Verification items for the finished model (mm, model axes). Face numbers are marked on the shaded views. A direction names the side the tool comes from. Coordinates: 2 decimals unless noted, no trailing zeros. Write each loop counter-clockwise with the first axis right and the second up, starting at its lowest first coordinate (ties: lowest second). Pieces come first, ordered by that corner, then holes. Notation, with made-up numbers: (18.5, -34) -> (41.5, -34) arc R38 cw to (41.5, 5) -> close; hole circle Ø2 at (19, 59.5). An arc over 180 degrees is marked (long way). Use CSV: the item, a comma, the result in double quotes.
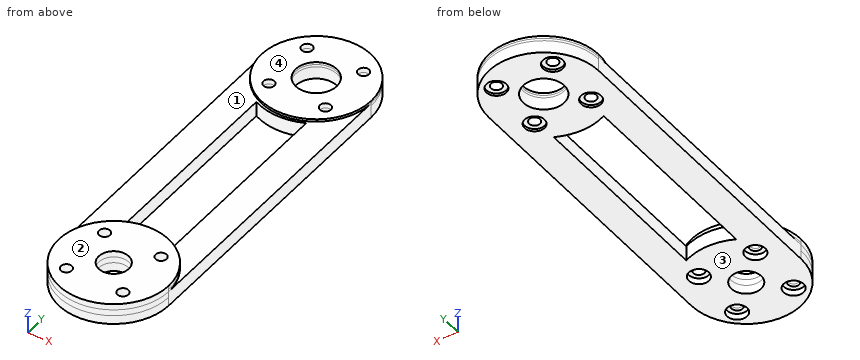
```python
from build123d import *

# Parameters (mm, degrees)
BOSS_EXTRUDE1_DEPTH           = 3
BOSS_EXTRUDE2_START           = -0.5
SKETCH1_3_R                   = 11
BOSS_EXTRUDE2_DEPTH           = 0.5
SKETCH2_R                     = 4.1
SKETCH2_R_2                   = 1.1000000000000099
CUT_EXTRUDE1_DEPTH            = 3.5
SKETCH2_3_R                   = 2.000000000000007
CUT_EXTRUDE2_DEPTH            = 0.5
CIRPATTERN2_COUNT             = 4
BOSS_EXTRUDE3_START           = -1.225
SKETCH1_5_R                   = 11
BOSS_EXTRUDE3_DEPTH           = 1.225
SKETCH3_R                     = 3.0000000000000004
SKETCH3_R_2                   = 1.1
CUT_EXTRUDE3_DEPTH            = 4.225
SKETCH3_3_R                   = 2.0000000000000027
CUT_EXTRUDE4_DEPTH            = 1.225
CIRPATTERN3_COUNT             = 4
BODY_MOVE_COPY1_START         = -3
BODY_MOVE_COPY1_OUTLINE_R     = 2
BODY_MOVE_COPY1_OUTLINE_R_2   = 3
BODY_MOVE_COPY1_OUTLINE_R_3   = 4.1
BODY_MOVE_COPY1_DEPTH         = 3
BODY_MOVE_COPY1_START_2       = -2.5
BODY_MOVE_COPY1_2_OUTLINE_R   = 2
BODY_MOVE_COPY1_2_OUTLINE_R_2 = 1.1
BODY_MOVE_COPY1_2_DEPTH       = 2
BODY_MOVE_COPY1_START_3       = -1.775
BODY_MOVE_COPY1_3_OUTLINE_R   = 2
BODY_MOVE_COPY1_3_OUTLINE_R_2 = 1.1
BODY_MOVE_COPY1_3_DEPTH       = 0.55
BODY_MOVE_COPY1_START_4       = 0.5
BODY_MOVE_COPY1_4_OUTLINE_R   = 4.1
BODY_MOVE_COPY1_4_OUTLINE_R_2 = 1.1
BODY_MOVE_COPY1_4_DEPTH       = 2.5
BODY_MOVE_COPY1_START_5       = 1.225
BODY_MOVE_COPY1_5_OUTLINE_R   = 11
BODY_MOVE_COPY1_5_OUTLINE_R_2 = 3
BODY_MOVE_COPY1_5_OUTLINE_R_3 = 1.1
BODY_MOVE_COPY1_5_DEPTH       = 1.775
BODY_MOVE_COPY1_6_DEPTH       = 0.5


# Read off the part's stored shape, not the designer's step: Body-Move/Copy1
with BuildPart() as part:
    # Sketch1 → Boss-Extrude1 (new body)
    with BuildSketch(Plane.XY):
        with BuildLine():
            Line((-11.000000000000004, 30), (-11, -30))
            ThreePointArc((-11, -30), (-2.02e-15, -41), (11, -30.000000000000004))
            Line((11, -30), (10.999999999999996, 30))
            ThreePointArc((10.999999999999996, 30), (-5.6e-16, 41), (-11.000000000000004, 30.000000000000007))
        make_face()
        with BuildLine():
            ThreePointArc((4.999999999999998, -19.643842411396), (2.89e-15, -18.49999999999999), (-4.999999999999995, -19.643842411396))
            Line((-4.999999999999993, -19.643842411396008), (-5.0000000000000036, 19.643842411396008))
            ThreePointArc((-5.000000000000004, 19.643842411396008), (1.78e-15, 18.5), (5.000000000000006, 19.643842411396008))
            Line((5.0000000000000036, 19.643842411396008), (4.999999999999998, -19.643842411396008))
        make_face(mode=Mode.SUBTRACT)
    extrude(amount=BOSS_EXTRUDE1_DEPTH)

    # Sketch1<3> → Boss-Extrude2 (add)
    with BuildSketch(Plane.XY.offset(BOSS_EXTRUDE2_START)):
        with Locations((-3.67e-15, 30)):
            Circle(SKETCH1_3_R)
    extrude(amount=BOSS_EXTRUDE2_DEPTH)

    # Sketch2 → Cut-Extrude1 (cut)
    with BuildSketch(Plane.XY.offset(3)):
        with Locations((-3.67e-15, 30)):
            Circle(SKETCH2_R)
        with Locations((5.6568542494923415, 35.656854249492405)):
            Circle(SKETCH2_R_2)
    cut_extrude1 = extrude(amount=-CUT_EXTRUDE1_DEPTH, mode=Mode.SUBTRACT)

    # Sketch2<3> → Cut-Extrude2 (cut)
    with BuildSketch(Plane.XY.offset(3)):
        with Locations((5.6568542494923415, 35.656854249492405)):
            Circle(SKETCH2_3_R)
    cut_extrude2 = extrude(amount=-CUT_EXTRUDE2_DEPTH, mode=Mode.SUBTRACT)

    # CirPattern2: Cut-Extrude1, Cut-Extrude2 ×4 about axis
    cirpattern2_axis = Axis((-1.339e-14, 30.00000000000001, 0), (0, 0, 1))
    add([cut_extrude1.rotate(cirpattern2_axis, i * 360 / CIRPATTERN2_COUNT) for i in range(1, CIRPATTERN2_COUNT)], mode=Mode.SUBTRACT)
    add([cut_extrude2.rotate(cirpattern2_axis, i * 360 / CIRPATTERN2_COUNT) for i in range(1, CIRPATTERN2_COUNT)], mode=Mode.SUBTRACT)

    # Sketch1<5> → Boss-Extrude3 (add)
    with BuildSketch(Plane.XY.offset(BOSS_EXTRUDE3_START)):
        with Locations((0, -30)):
            Circle(SKETCH1_5_R)
    extrude(amount=BOSS_EXTRUDE3_DEPTH)

    # Sketch3 → Cut-Extrude3 (cut)
    with BuildSketch(Plane.XY.offset(3)):
        with Locations((0, -30)):
            Circle(SKETCH3_R)
        with Locations((5.656854249492389, -24.34314575050763)):
            Circle(SKETCH3_R_2)
    cut_extrude3 = extrude(amount=-CUT_EXTRUDE3_DEPTH, mode=Mode.SUBTRACT)

    # Sketch3<3> → Cut-Extrude4 (cut)
    with BuildSketch(Plane.XY.offset(3)):
        with Locations((5.656854249492389, -24.34314575050763)):
            Circle(SKETCH3_3_R)
    cut_extrude4 = extrude(amount=-CUT_EXTRUDE4_DEPTH, mode=Mode.SUBTRACT)

    # CirPattern3: Cut-Extrude3, Cut-Extrude4 ×4 about axis
    cirpattern3_axis = Axis((-9.49e-15, -29.99999999999999, 0), (0, 0, 1))
    add([cut_extrude3.rotate(cirpattern3_axis, i * 360 / CIRPATTERN3_COUNT) for i in range(1, CIRPATTERN3_COUNT)], mode=Mode.SUBTRACT)
    add([cut_extrude4.rotate(cirpattern3_axis, i * 360 / CIRPATTERN3_COUNT) for i in range(1, CIRPATTERN3_COUNT)], mode=Mode.SUBTRACT)

    # Body-Move/Copy1 outline → Body-Move/Copy1 (add)
    with BuildSketch(Plane.XY.offset(BODY_MOVE_COPY1_START)):
        with BuildLine():
            Line((-11, 30), (-11, -30))
            ThreePointArc((-11, -30), (0, -41), (11, -30))
            Line((11, -30), (11, 30))
            ThreePointArc((11, 30), (0, 41), (-11, 30))
        make_face()
        with BuildLine():
            Line((-5, -19.643842411), (-5, 19.643842411))
            ThreePointArc((-5, 19.643842411), (0, 18.5), (5, 19.643842411))
            Line((5, 19.643842411), (5, -19.643842411))
            ThreePointArc((5, -19.643842411), (0, -18.5), (-5, -19.643842411))
        make_face(mode=Mode.SUBTRACT)
        with Locations((5.656854249, -24.343145751)):
            Circle(BODY_MOVE_COPY1_OUTLINE_R, mode=Mode.SUBTRACT)
        with Locations((-5.656854249, -35.656854249)):
            Circle(BODY_MOVE_COPY1_OUTLINE_R, mode=Mode.SUBTRACT)
        with Locations((-5.656854249, -24.343145751)):
            Circle(BODY_MOVE_COPY1_OUTLINE_R, mode=Mode.SUBTRACT)
        with Locations((0, -30)):
            Circle(BODY_MOVE_COPY1_OUTLINE_R_2, mode=Mode.SUBTRACT)
        with Locations((5.656854249, -35.656854249)):
            Circle(BODY_MOVE_COPY1_OUTLINE_R, mode=Mode.SUBTRACT)
        with Locations((5.656854249, 35.656854249)):
            Circle(BODY_MOVE_COPY1_OUTLINE_R, mode=Mode.SUBTRACT)
        with Locations((-5.656854249, 24.343145751)):
            Circle(BODY_MOVE_COPY1_OUTLINE_R, mode=Mode.SUBTRACT)
        with Locations((-5.656854249, 35.656854249)):
            Circle(BODY_MOVE_COPY1_OUTLINE_R, mode=Mode.SUBTRACT)
        with Locations((0, 30)):
            Circle(BODY_MOVE_COPY1_OUTLINE_R_3, mode=Mode.SUBTRACT)
        with Locations((5.656854249, 24.343145751)):
            Circle(BODY_MOVE_COPY1_OUTLINE_R, mode=Mode.SUBTRACT)
    extrude(amount=BODY_MOVE_COPY1_DEPTH)

    # Body-Move_Copy1 2 outline → Body-Move_Copy1 2 (add)
    # profile 1 of 4: a face of its own
    with BuildSketch(Plane.XY.offset(BODY_MOVE_COPY1_START_2)):
        with Locations((5.656854249, 35.656854249)):
            Circle(BODY_MOVE_COPY1_2_OUTLINE_R)
        with Locations((5.656854249, 35.656854249)):
            Circle(BODY_MOVE_COPY1_2_OUTLINE_R_2, mode=Mode.SUBTRACT)
    # profile 2 of 4: a face of its own
    with BuildSketch(Plane.XY.offset(BODY_MOVE_COPY1_START_2)):
        with Locations((5.656854249, 24.343145751)):
            Circle(BODY_MOVE_COPY1_2_OUTLINE_R)
        with Locations((5.656854249, 24.343145751)):
            Circle(BODY_MOVE_COPY1_2_OUTLINE_R_2, mode=Mode.SUBTRACT)
    # profile 3 of 4: a face of its own
    with BuildSketch(Plane.XY.offset(BODY_MOVE_COPY1_START_2)):
        with Locations((-5.656854249, 35.656854249)):
            Circle(BODY_MOVE_COPY1_2_OUTLINE_R)
        with Locations((-5.656854249, 35.656854249)):
            Circle(BODY_MOVE_COPY1_2_OUTLINE_R_2, mode=Mode.SUBTRACT)
    # profile 4 of 4: a face of its own
    with BuildSketch(Plane.XY.offset(BODY_MOVE_COPY1_START_2)):
        with Locations((-5.656854249, 24.343145751)):
            Circle(BODY_MOVE_COPY1_2_OUTLINE_R)
        with Locations((-5.656854249, 24.343145751)):
            Circle(BODY_MOVE_COPY1_2_OUTLINE_R_2, mode=Mode.SUBTRACT)
    extrude(amount=BODY_MOVE_COPY1_2_DEPTH)

    # Body-Move_Copy1 3 outline → Body-Move_Copy1 3 (add)
    # profile 1 of 4: a face of its own
    with BuildSketch(Plane.XY.offset(BODY_MOVE_COPY1_START_3)):
        with Locations((5.656854249, -24.343145751)):
            Circle(BODY_MOVE_COPY1_3_OUTLINE_R)
        with Locations((5.656854249, -24.343145751)):
            Circle(BODY_MOVE_COPY1_3_OUTLINE_R_2, mode=Mode.SUBTRACT)
    # profile 2 of 4: a face of its own
    with BuildSketch(Plane.XY.offset(BODY_MOVE_COPY1_START_3)):
        with Locations((5.656854249, -35.656854249)):
            Circle(BODY_MOVE_COPY1_3_OUTLINE_R)
        with Locations((5.656854249, -35.656854249)):
            Circle(BODY_MOVE_COPY1_3_OUTLINE_R_2, mode=Mode.SUBTRACT)
    # profile 3 of 4: a face of its own
    with BuildSketch(Plane.XY.offset(BODY_MOVE_COPY1_START_3)):
        with Locations((-5.656854249, -24.343145751)):
            Circle(BODY_MOVE_COPY1_3_OUTLINE_R)
        with Locations((-5.656854249, -24.343145751)):
            Circle(BODY_MOVE_COPY1_3_OUTLINE_R_2, mode=Mode.SUBTRACT)
    # profile 4 of 4: a face of its own
    with BuildSketch(Plane.XY.offset(BODY_MOVE_COPY1_START_3)):
        with Locations((-5.656854249, -35.656854249)):
            Circle(BODY_MOVE_COPY1_3_OUTLINE_R)
        with Locations((-5.656854249, -35.656854249)):
            Circle(BODY_MOVE_COPY1_3_OUTLINE_R_2, mode=Mode.SUBTRACT)
    extrude(amount=BODY_MOVE_COPY1_3_DEPTH)

    # Body-Move_Copy1 4 outline → Body-Move_Copy1 4 (cut)
    with BuildSketch(Plane.XY.offset(BODY_MOVE_COPY1_START_4)):
        with BuildLine():
            ThreePointArc((-11, -30), (0, -19), (11, -30))
            Line((11, -30), (11, 30))
            ThreePointArc((11, 30), (0, 41), (-11, 30))
            Line((-11, 30), (-11, -30))
        make_face()
        with BuildLine():
            Line((-5, -19.643842411), (-5, 19.643842411))
            ThreePointArc((-5, 19.643842411), (0, 18.5), (5, 19.643842411))
            Line((5, 19.643842411), (5, -19.643842411))
            ThreePointArc((5, -19.643842411), (0, -18.5), (-5, -19.643842411))
        make_face(mode=Mode.SUBTRACT)
        with Locations((0, 30)):
            Circle(BODY_MOVE_COPY1_4_OUTLINE_R, mode=Mode.SUBTRACT)
        with Locations((5.656854249, 35.656854249)):
            Circle(BODY_MOVE_COPY1_4_OUTLINE_R_2, mode=Mode.SUBTRACT)
        with Locations((-5.656854249, 24.343145751)):
            Circle(BODY_MOVE_COPY1_4_OUTLINE_R_2, mode=Mode.SUBTRACT)
        with Locations((-5.656854249, 35.656854249)):
            Circle(BODY_MOVE_COPY1_4_OUTLINE_R_2, mode=Mode.SUBTRACT)
        with Locations((5.656854249, 24.343145751)):
            Circle(BODY_MOVE_COPY1_4_OUTLINE_R_2, mode=Mode.SUBTRACT)
    extrude(amount=BODY_MOVE_COPY1_4_DEPTH, mode=Mode.SUBTRACT)

    # Body-Move_Copy1 5 outline → Body-Move_Copy1 5 (cut)
    with BuildSketch(Plane.XY.offset(BODY_MOVE_COPY1_START_5)):
        with Locations((0, -30)):
            Circle(BODY_MOVE_COPY1_5_OUTLINE_R)
        with Locations((0, -30)):
            Circle(BODY_MOVE_COPY1_5_OUTLINE_R_2, mode=Mode.SUBTRACT)
        with Locations((-5.656854249, -35.656854249)):
            Circle(BODY_MOVE_COPY1_5_OUTLINE_R_3, mode=Mode.SUBTRACT)
        with Locations((-5.656854249, -24.343145751)):
            Circle(BODY_MOVE_COPY1_5_OUTLINE_R_3, mode=Mode.SUBTRACT)
        with Locations((5.656854249, -35.656854249)):
            Circle(BODY_MOVE_COPY1_5_OUTLINE_R_3, mode=Mode.SUBTRACT)
        with Locations((5.656854249, -24.343145751)):
            Circle(BODY_MOVE_COPY1_5_OUTLINE_R_3, mode=Mode.SUBTRACT)
    extrude(amount=BODY_MOVE_COPY1_5_DEPTH, mode=Mode.SUBTRACT)

    # Body-Move_Copy1 6 outline → Body-Move_Copy1 6 (cut)
    with BuildSketch(Plane.XY):
        with BuildLine():
            ThreePointArc((-11, -30), (0, -19), (11, -30))
            Line((11, -30), (11, 30))
            ThreePointArc((11, 30), (0, 19), (-11, 30))
            Line((-11, 30), (-11, -30))
        make_face()
        with BuildLine():
            Line((-5, -19.643842411), (-5, 19.643842411))
            ThreePointArc((-5, 19.643842411), (0, 18.5), (5, 19.643842411))
            Line((5, 19.643842411), (5, -19.643842411))
            ThreePointArc((5, -19.643842411), (0, -18.5), (-5, -19.643842411))
        make_face(mode=Mode.SUBTRACT)
    extrude(amount=BODY_MOVE_COPY1_6_DEPTH, mode=Mode.SUBTRACT)


solid = part.part
```
1) Cross-section at B-B (y = -7.5). Record the boundary of the cut face in (x, z).
Return value:
outline,"(-11, -3) -> (-5, -3) -> (-5, 0) -> (-11, 0) -> close; (5, -3) -> (11, -3) -> (11, 0) -> (5, 0) -> close"
2) Cross-section at C-C (x = 8.5). Record the boundary of the cut face in (y, z) (3 decimals).
Return value:
outline,"(-36.982, -3) -> (36.982, -3) -> (36.982, 0.5) -> (23.018, 0.5) -> (23.018, 0) -> (-23.018, 0) -> (-23.018, 1.225) -> (-36.982, 1.225) -> close"
3) Gauge pin test, flat ends, axial feed: pin 1 (1 mm diameter, centred on x = -8, y = 5, fed in from +Z); pin 2 (2 mm diameter, centred on x = -4.5, z = -1.5, fed in from +Y); pin 3 (2.5 mm diameter, centred on x = 5.66, y = -24.34, fed in from -Z) (3 decimals); pin 4 (2 mm diameter, centred on x = 5.66, y = 24.34, fed in from +Z). Record the tip position at first contact, or that the pin passes through.
Return value:
pin 1,"z = 0"
pin 2,"y = 40.43"
pin 3,"z = -1.775"
pin 4,"through"
4) Set-up check for the marked faces 3 and 4: record each of +Z, -Z, +X, -X, +Y, -Y from which the full face is reachable in a straight line by a thin tool's end or side.
Return value:
face 3,"-Z, +X, -X, +Y, -Y"
face 4,"+Z, +X, -X, +Y"
5) Cross-section at A-A (x = 0). Record the boundary of the cut face in (y, z) (3 decimals).
Return value:
outline,"(-41, -3) -> (-33, -3) -> (-33, 1.225) -> (-41, 1.225) -> close; (-27, -3) -> (-18.5, -3) -> (-18.5, 0) -> (-19, 0) -> (-19, 1.225) -> (-27, 1.225) -> close; (18.5, -3) -> (25.9, -3) -> (25.9, 0.5) -> (19, 0.5) -> (19, 0) -> (18.5, 0) -> close; (34.1, -3) -> (41, -3) -> (41, 0.5) -> (34.1, 0.5) -> close"
6) Scan lines: L1, parallel to X at y = -11, z = -1.8; L2, parallel to X at y = 19.5, z = -2.2; L3, parallel to Y at x = -5.5, z = -2.3. Record each from-to range of solid material in increasing order.
Return value:
L1,"-11 to -5, 5 to 11"
L2,"-11 to -5, -4.69 to 4.69, 5 to 11"
L3,"-39.53 to -37.65, -33.66 to -26.34, -22.35 to 23.25, 25.43 to 34.57, 36.75 to 39.53"
7) Mould release check, pull along Y, two halves, no side actions. Record for the marked faces 1 and 2: released by +Y, released by -Y, zero draft, split by the parting line, or undercut.
Return value:
face 1,"undercut"
face 2,"zero draft"
